The listing builds one solid part. Answer for the finished solid, in the listing's coordinates (mm). Coordinates: 2 decimals unless noted, no trailing zeros. Order: outer loops, then holes, each group sorted by start corner. A loop starts at its lowest first (then second) coordinate and runs counter-clockwise, first axis right, second up. Notation, with made-up numbers: (-1, 68) -> (56, 68) arc R24 ccw to (56, 107) -> close; hole circle Ø8 at (-17.75, 67). An arc over 180 degrees is marked (long way). Answer in a Markdown table with one row per item.
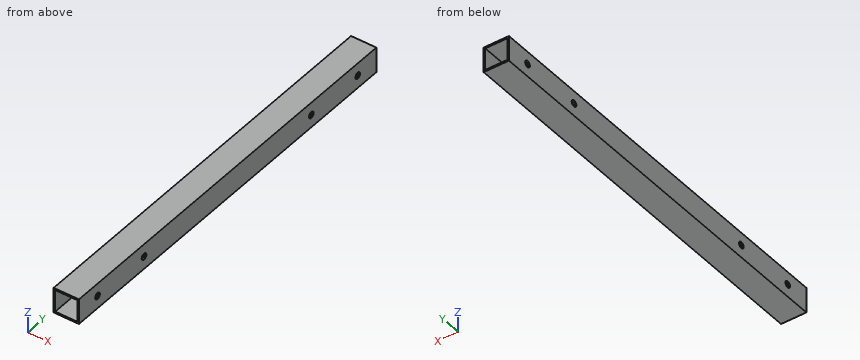
```python
from build123d import *

# Parameters (mm, degrees)
SKETCH1_W           = 50.8
SKETCH1_H           = 50.8
SKETCH1_W_2         = 44.416753927
SKETCH1_H_2         = 44.416753927
BOSS_EXTRUDE1_DEPTH = 812.8
SKETCH2_R           = 6.35
CUT_EXTRUDE1_DEPTH  = 51.8


with BuildPart() as part:
    # Sketch1 → Boss-Extrude1 (new body)
    with BuildSketch(Plane(origin=(0, 0, 0), x_dir=(1, 0, 0), z_dir=(0, 1, 0))):
        Rectangle(SKETCH1_W, SKETCH1_H)
        with Locations((-0.016623037, 0.016623037)):
            Rectangle(SKETCH1_W_2, SKETCH1_H_2, mode=Mode.SUBTRACT)
    extrude(amount=BOSS_EXTRUDE1_DEPTH)

    # Sketch2 → Cut-Extrude1 (cut, through all)
    with BuildSketch(Plane.ZY.offset(25.4)):
        with Locations((0, 50.8)):
            Circle(SKETCH2_R)
        with Locations((0, 177.8)):
            Circle(SKETCH2_R)
        with Locations((0, 635)):
            Circle(SKETCH2_R)
        with Locations((0, 762)):
            Circle(SKETCH2_R)
    extrude(amount=-CUT_EXTRUDE1_DEPTH, mode=Mode.SUBTRACT)


solid = part.part
```
(1) A cutting plane is placed at B-B, the plane z = 14. Determine the outline of the cut face in (x, y) (3 decimals).
Check values:
| item | result |
|---|---|
| outline | (-25.4, 0) -> (-22.225, 0) -> (-22.225, 812.8) -> (-25.4, 812.8) -> close; (22.192, 0) -> (25.4, 0) -> (25.4, 812.8) -> (22.192, 812.8) -> close |
(2) A cutting plane is placed at C-C, the plane y = 143. Determine the outline of the cut face in (x, z) (3 decimals).
Check values:
| item | result |
|---|---|
| outline | (-25.4, -25.4) -> (25.4, -25.4) -> (25.4, 25.4) -> (-25.4, 25.4) -> close; hole (-22.225, -22.225) -> (22.192, -22.225) -> (22.192, 22.192) -> (-22.225, 22.192) -> close |
(3) A cutting plane is placed at A-A, the plane x = 2. Determine the outline of the cut face in (y, z) (3 decimals), then the cut area to 3 significant figures.
Check values:
| item | result |
|---|---|
| outline | (0, -25.4) -> (812.8, -25.4) -> (812.8, -22.225) -> (0, -22.225) -> close; (0, 22.192) -> (812.8, 22.192) -> (812.8, 25.4) -> (0, 25.4) -> close |
| area | 5,190 mm² |
(4) Find the intervals of material crossed by line 1 along Y through (x, z) = (24.1, 0); line 2 along Z through (x, y) = (16, 325.5) (3 decimals), in increasing order. Write a range as from..to.
Check values:
| item | result |
|---|---|
| line 1 | 0..44.45, 57.15..171.45, 184.15..628.65, 641.35..755.65, 768.35..812.8 |
| line 2 | -25.4..-22.225, 22.192..25.4 |
